Can you work these out from the model? Positions are in its coordinate system, mm. A direction names the side the tool comes from. Give positions to 0.01 mm unless a question says otherwise; leave off trailing zeros. Loops run counter-clockwise (first coordinate to the right, second up) from the corner with the lowest first, then second, coordinate; pieces in that order, holes last. Notation, with made-up numbers: M 52,1.25 L 86,1.25 A10 cw 86,20.25 Z; hole C 51,8.5 d3. An arc over 180 degrees is marked long. Answer as a JSON object with one key per item and string values.
Autodesk Inventor part; units mm, degrees
ref_plane "YZ Plane" through (0, 0, 0) normal (1, 0, 0) x (0, 1, 0)
ref_plane "XZ Plane" through (0, 0, 0) normal (0, 1, 0) x (-1, 0, 0)
ref_plane "XY Plane" through (0, 0, 0) normal (0, 0, 1) x (1, 0, 0)
sketch "Sketch1" plane through (0, 0, 0) normal (0, 0, 1) x (1, 0, 0)
  line L0 (0, 0) -> (25.4, 0)
  line L1 (25.4, 0) -> (25.4, 25.4)
  line L2 (25.4, 25.4) -> (0, 25.4)
  line L3 (0, 25.4) -> (0, 0)
  dimension "d0" = 25.4
  dimension "d1" = 25.4
extrude "Extrusion1" add sketch "Sketch1" along normal blind 660.4
shell "Shell1" thickness 1.5875 removed faces 2 at (8.4667, 16.9333, 0) at (8.4667, 16.9333, 660.4)
equation "\"d1\" = d0"
properties part number "CrossFrameRail" material "Aluminum-6061"
1) Please list where this line runs through material, in increasing order: line 1 along Y through (x, z) = (20.75, 178). Write a range as from..to.
Answer list:
{"line 1": "0..1.59, 23.81..25.4"}
2) Suppose I cut it at C-C, the plane z = 181. Write out the boundary of the cut face in (x, y), and give its area (3 significant figures).
Answer list:
{"outline": "M 0,0 L 25.4,0 L 25.4,25.4 L 0,25.4 Z; hole M 1.59,1.59 L 23.81,1.59 L 23.81,23.81 L 1.59,23.81 Z", "area": "151 mm^2"}
3) For faces 4 (the flat face through (1.588, 13, 326)), 5 (the flat face through (0, 13, 326)), which set-ups out of +Z, -Z, +X, -X, +Y, -Y let a thin tool reach every point of the face, with its end or its side?
Answer list:
{"face 4": "+Z, -Z", "face 5": "+Z, -Z, -X, +Y, -Y"}
4) Suppose I cut it at A-A, the plane y = 13.75. Write out the boundary of the cut face in (x, z).
Answer list:
{"outline": "M 0,0 L 1.59,0 L 1.59,660.4 L 0,660.4 Z; M 23.81,0 L 25.4,0 L 25.4,660.4 L 23.81,660.4 Z"}
5) If we mould it in two halves opening along Y, with no side actions, what happens to faces 1 (the flat face through (13, 0, 326)), 2 (the flat face through (23.812, 13, 326)), 3 (the flat face through (1, 13, 0))? For each: +Y half, -Y half, draft (parallel to the pull), parting line (faces both ways), or undercut.
Answer list:
{"face 1": "-Y half", "face 2": "undercut", "face 3": "draft"}
